from build123d import *

# Parameters (mm, degrees)
F1_DEPTH = 25
F2_SIZE2 = 13
F2_SIZE  = 8
F3_SIZE  = 1.5


with BuildPart() as f1:
    # F0 (on Top) → F1 (new body)
    with BuildSketch(Plane.XY):
        Polygon((0, 18), (0, 0), (18, 0), (18, 3), (3, 3), (3, 18), align=None)
    extrude(amount=F1_DEPTH)

    # F2
    f2_edges = [f1.edges().sort_by_distance(p)[0] for p in [
        (1.5, 18, 25),
        (18, 1.5, 25),
    ]]
    chamfer(f2_edges, length=F2_SIZE, length2=F2_SIZE2)

    # F3
    f3_edges = [f1.edges().sort_by_distance(p)[0] for p in [
        (0, 18, 8.5),
        (0, 0, 12.5),
        (18, 0, 8.5),
    ]]
    chamfer(f3_edges, length=F3_SIZE)


solid = f1.part
Could you check a few things on this model? Use its own coordinates, in mm. A direction names the side the tool comes from. Give positions to 0.01 mm unless a question says otherwise; leave off trailing zeros. Order: outer loops, then holes, each group sorted by start corner. A loop starts at its lowest first (then second) coordinate and runs counter-clockwise, first axis right, second up. Notation, with made-up numbers: (-13, -16.5) - (-7, -16.5) arc R11 ccw to (-7, -7.5) - close; hole circle Ø8 at (64, -7). An arc over 180 degrees is marked (long way). One line per item, written item: value. Start each with the question number.
1. For faces 1 (the face through (9, 0, 12)), 2 (the face through (3, 10, 10)), which set-ups out of +Z, -Z, +X, -X, +Y, -Y let a thin tool reach every point of the face, with its end or its side?
2. Imagine slicing it at A-A on z = 14.5. List the corners of the cut face in (x, y) for me.
3. For P1, Ø4.5, axis at x = 7.5, z = 17, coming from the +Y side; P2, Ø3, axis at y = 15.5, z = 4.5, coming from the +X side, each with a flat end and sliding along its axis, tell me the tip position at first contact or that it passes through.
4. If I drill on probe 1 along X at (y, z) = (11, 14.75); probe 2 along Z at (x, y) = (1, 16.5), over which ranges is the centre line in solid material (lowest first)?
5. Imagine slicing it at D-D on z = 21.5. List the corners of the cut face in (x, y) for me, plus the area to 3 significant figures.
6. Imagine slicing it at B-B on x = 2. List the corners of the cut face in (y, z) for me.
7. Imagine slicing it at C-C on y = 5.5. List the corners of the cut face in (x, z) for me, plus the area to 3 significant figures.
Values:
1. face 1: +Z, -Z, +X, -X, -Y
1. face 2: +Z, -Z, +X, +Y
2. outline: (0, 1.5) - (1.5, 0) - (16.5, 0) - (18, 1.5) - (18, 3) - (3, 3) - (3, 18) - (1.5, 18) - (0, 16.5) - close
3. P1: y = 3
3. P2: x = 3
4. probe 1: 0 to 3
4. probe 2: 0 to 17.92
5. outline: (0, 1.5) - (1.5, 0) - (10.69, 0) - (10.69, 3) - (3, 3) - (3, 10.69) - (0, 10.69) - close
5. area: 54.0 mm²
6. outline: (0, 0) - (18, 0) - (18, 17) - (5, 25) - (0, 25) - close
7. outline: (0, 0) - (3, 0) - (3, 24.69) - (0, 24.69) - close
7. area: 74.1 mm²
